Input: part model. Units: mm. Frame: model coordinates. Coordinates: 2 decimals unless noted, no trailing zeros. Order: outer loops, then holes, each group sorted by start corner. A loop starts at its lowest first (then second) coordinate and runs counter-clockwise, first axis right, second up. Notation, with made-up numbers: (-38, -9) - (-11, -9) arc R20 ccw to (-11, 0) - close; hole circle Ø4 at (76.5, 26.25). An arc over 180 degrees is marked (long way). Answer as CSV lines item,"result". Start each with the question number.
Item 1: Material intervals for line 1 along X through (y, z) = (1.55, -5); line 2 along X through (y, z) = (2.65, -6); line 3 along Z through (x, y) = (432, 2.5), sorted ascending.
Item 2: First-contact query: pin 1 (0.9 mm diameter, centred on x = 439, y = 1.5, fed in from +Z); pin 2 (1.6 mm diameter, centred on x = 131.5, y = 1, fed in from -Z). Flat tips, straight axial feed; report the tip coordinate or a pass-through.
Item 3: Section A-A (x = 144). Output: boundary loops of the cut face in (y, z) (3 decimals).
Item 4: Section B-B (y = 1.6). State how many separate pieces and enclosed holes the cut face has, and give its area (3 significant figures).
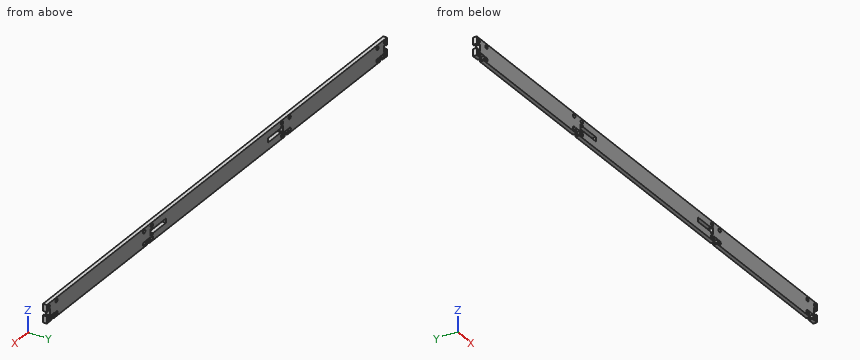
from build123d import *

# Parameters (mm, degrees)
SKETCH1_R           = 1.5
BOSS_EXTRUDE1_DEPTH = 3.175
CUT_EXTRUDE19_DEPTH = 445.76435404


with BuildPart() as part:
    # Sketch1 → Boss-Extrude1 (new body)
    with BuildSketch(Plane(origin=(0, 0, 0), x_dir=(1, 0, 0), z_dir=(0, 1, 0))):
        Polygon((0, 7.5), (0, 0), (444.5, 0), (444.5, 15), (0, 15), align=None)
        with Locations(Location((2.5, 2.5, 0), (0, 0, 270))):
            Circle(SKETCH1_R, mode=Mode.SUBTRACT)
        with Locations(Location((12.5, 2.5, 0), (0, 0, 270))):
            Circle(SKETCH1_R, mode=Mode.SUBTRACT)
        with Locations(Location((127.2, 2.5, 0), (0, 0, 270))):
            Circle(SKETCH1_R, mode=Mode.SUBTRACT)
        with Locations(Location((137.2, 2.5, 0), (0, 0, 270))):
            Circle(SKETCH1_R, mode=Mode.SUBTRACT)
        with Locations(Location((2.5, 12.5, 0), (0, 0, 270))):
            Circle(SKETCH1_R, mode=Mode.SUBTRACT)
        with Locations(Location((12.5, 12.5, 0), (0, 0, 270))):
            Circle(SKETCH1_R, mode=Mode.SUBTRACT)
        with Locations(Location((127.2, 12.5, 0), (0, 0, 270))):
            Circle(SKETCH1_R, mode=Mode.SUBTRACT)
        with Locations(Location((137.2, 12.5, 0), (0, 0, 270))):
            Circle(SKETCH1_R, mode=Mode.SUBTRACT)
        with Locations(Location((442, 12.5, 0), (0, 0, 270))):
            Circle(SKETCH1_R, mode=Mode.SUBTRACT)
        with Locations(Location((307.3, 2.5, 0), (0, 0, 270))):
            Circle(SKETCH1_R, mode=Mode.SUBTRACT)
        with Locations(Location((317.3, 2.5, 0), (0, 0, 270))):
            Circle(SKETCH1_R, mode=Mode.SUBTRACT)
        with Locations(Location((432, 2.5, 0), (0, 0, 270))):
            Circle(SKETCH1_R, mode=Mode.SUBTRACT)
        with Locations(Location((442, 2.5, 0), (0, 0, 270))):
            Circle(SKETCH1_R, mode=Mode.SUBTRACT)
        with Locations(Location((307.3, 12.5, 0), (0, 0, 270))):
            Circle(SKETCH1_R, mode=Mode.SUBTRACT)
        with Locations(Location((317.3, 12.5, 0), (0, 0, 270))):
            Circle(SKETCH1_R, mode=Mode.SUBTRACT)
        with Locations(Location((432, 12.5, 0), (0, 0, 270))):
            Circle(SKETCH1_R, mode=Mode.SUBTRACT)
    extrude(amount=BOSS_EXTRUDE1_DEPTH)

    # Sketch23 → Cut-Extrude19 (cut, through all)
    with BuildSketch(Plane(origin=(0, 3.175, 0), x_dir=(1, 0, 0), z_dir=(0, 1, 0))):
        Polygon((444.5, 7.5), (444.5, 9.25), (443.3, 9.25), (443.3, 10.35), (440.5, 10.35), (440.5, 4.65), (443.3, 4.65), (443.3, 5.75), (444.5, 5.75), align=None)
        Polygon((437, 15), (435.416405275, 15), (435.416405275, 13.8), (434.316405275, 13.8), (434.316405275, 11), (439.695743789, 11), (439.695743789, 13.8), (438.595743789, 13.8), (438.595743789, 15), align=None)
        Polygon((306, 5.75), (306, 4.65), (308.8, 4.65), (308.8, 10.35), (306, 10.35), (306, 9.25), (304.8, 9.25), (288.8, 9.25), (288.8, 5.75), (304.8, 5.75), align=None)
        Polygon((312.3, 15), (310.704256211, 15), (310.704256211, 13.8), (309.604256211, 13.8), (309.604256211, 11), (314.983594725, 11), (314.983594725, 13.8), (313.883594725, 13.8), (313.883594725, 15), align=None)
        Polygon((135.7, 4.65), (138.5, 4.65), (138.5, 5.75), (139.7, 5.75), (155.7, 5.75), (155.7, 9.25), (139.7, 9.25), (138.5, 9.25), (138.5, 10.35), (135.7, 10.35), align=None)
        Polygon((132.2, 15), (130.616405275, 15), (130.616405275, 13.8), (129.516405275, 13.8), (129.516405275, 11), (134.895743789, 11), (134.895743789, 13.8), (133.795743789, 13.8), (133.795743789, 15), align=None)
        Polygon((7.5, 15), (5.904256211, 15), (5.904256211, 13.8), (4.804256211, 13.8), (4.804256211, 11), (10.183594725, 11), (10.183594725, 13.8), (9.083594725, 13.8), (9.083594725, 15), align=None)
        Polygon((0, 9.25), (0, 7.5), (0, 5.75), (1.2, 5.75), (1.2, 4.65), (4, 4.65), (4, 10.35), (1.2, 10.35), (1.2, 9.25), align=None)
    extrude(amount=-CUT_EXTRUDE19_DEPTH, mode=Mode.SUBTRACT)


solid = part.part
Determined:
1,line 1,"x = 0 to 1.2, 4 to 135.7, 138.5 to 306, 308.8 to 440.5, 443.3 to 444.5"
1,line 2,"x = 4 to 135.7, 155.7 to 288.8, 308.8 to 440.5"
1,line 3,"z = -15 to -14, -11 to -4, -1 to 0"
2,pin 1,"stops at z = 0"
2,pin 2,"stops at z = -11"
3,outline,"(0, -15) - (3.175, -15) - (3.175, -9.25) - (0, -9.25) - close; (0, -5.75) - (3.175, -5.75) - (3.175, 0) - (0, 0) - close"
4,separate pieces,"1"
4,enclosed holes,"18"
4,area,"6,290 mm^2"
